The drawing under review shows one solid part. Ordinate dimensions are in mm from its lowest x, y, z. A direction names the side the tool comes from. Round coordinates to 2 decimals unless told otherwise and drop trailing zeros. Order: outer loops, then holes, each group sorted by start corner. A loop starts at its lowest first (then second) coordinate and runs counter-clockwise, first axis right, second up. Notation, with made-up numbers: (71.5, 64.5) - (120.5, 64.5) arc R26 ccw to (120.5, 99.5) - close; hole circle Ø1 at (57.25, 76). An arc over 180 degrees is marked (long way). One line per question, with ' | ' between items.
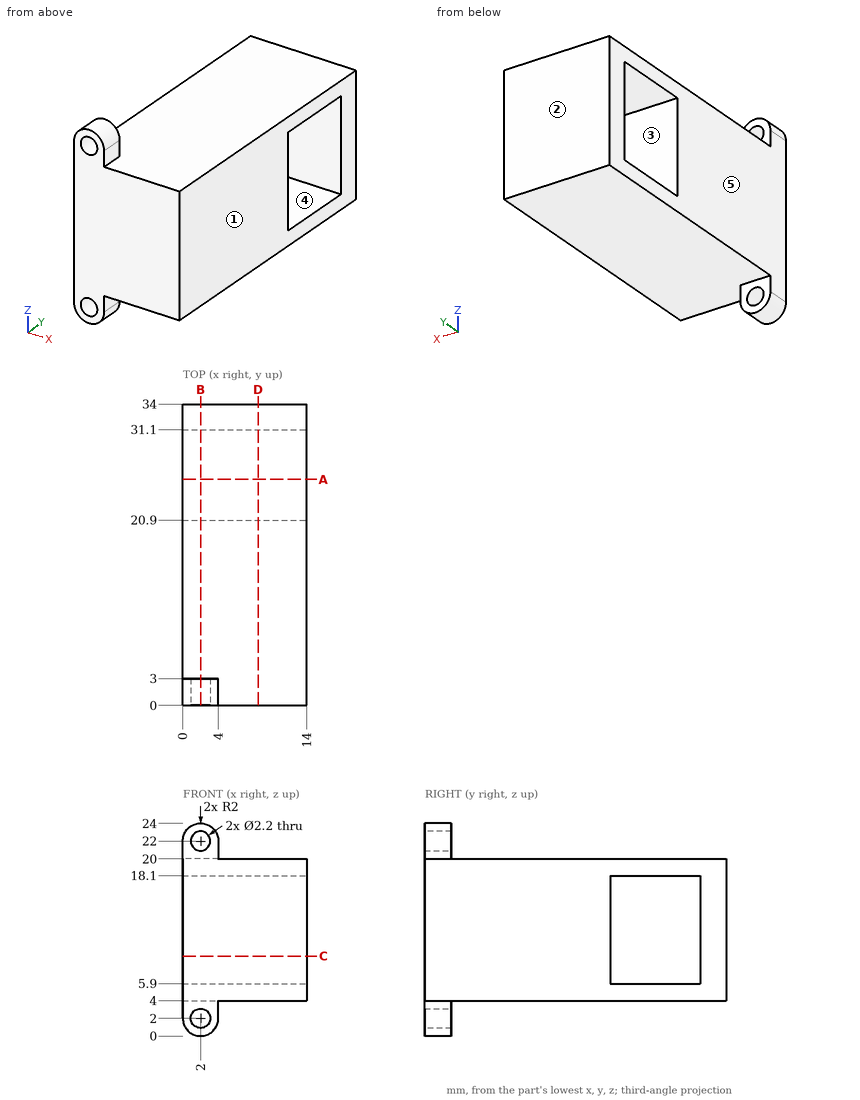
(1) We need section C-C on z = 9. State the section outline as (x, y) points.
Output values:
outline: (0, 0) - (14, 0) - (14, 20.9) - (0, 20.9) - close; (0, 31.1) - (14, 31.1) - (14, 34) - (0, 34) - close
(2) Insertion check: pin 1 (2 mm diameter, centred on x = 2.5, z = 2.5, fed in from +Y); pin 2 (0.6 mm diameter, centred on y = 2, z = 21, fed in from +X); pin 3 (1.5 mm diameter, centred on x = 5, y = 30.5, fed in from -Z); pin 4 (2.5 mm diameter, centred on x = 2, z = 2, fed in from -Y). Each pin has a flat end and moves straight along its axis. Give the tip position at first contact, or say it passes through.
Output values:
pin 1: y = 3 | pin 2: x = 4 | pin 3: z = 4 | pin 4: y = 0
(3) We need section D-D on x = 8.5. State the section outline as (y, z) points, plus the area to 3 significant figures.
Output values:
outline: (0, 4) - (34, 4) - (34, 20) - (0, 20) - close; hole (20.9, 5.9) - (31.1, 5.9) - (31.1, 18.1) - (20.9, 18.1) - close | area: 420 mm^2
(4) We need section A-A on y = 25.5. State the section outline as (x, z) points, plus the area to 3 significant figures.
Output values:
outline: (0, 4) - (14, 4) - (14, 5.9) - (0, 5.9) - close; (0, 18.1) - (14, 18.1) - (14, 20) - (0, 20) - close | area: 53.2 mm^2
(5) For probe 1 along Z at (x, y) = (13, 25.5); probe 2 along Y at (x, z) = (10.25, 14); probe 3 along X at (y, z) = (2.05, 22), list the stretches that pass through material, from the lowest coordinate up. Write a range as [from, to].
Output values:
probe 1: [4, 5.9], [18.1, 20] | probe 2: [0, 20.9], [31.1, 34] | probe 3: [0, 0.9], [3.1, 4]
(6) We need section B-B on x = 2. State the section outline as (y, z) points.
Output values:
outline: (0, 0) - (3, 0) - (3, 0.9) - (0, 0.9) - close; (0, 3.1) - (3, 3.1) - (3, 4) - (34, 4) - (34, 20) - (3, 20) - (3, 20.9) - (0, 20.9) - close; (0, 23.1) - (3, 23.1) - (3, 24) - (0, 24) - close; hole (20.9, 5.9) - (31.1, 5.9) - (31.1, 18.1) - (20.9, 18.1) - close
(7) For the marked faces 4 and 5, list the 3-axis set-ups (+Z, -Z, +X, -X, +Y, -Y) from which the entire face can be reached by the end or side of a thin tool; tool diameter is ignored.
Output values:
face 4: +X, -X | face 5: +Z, -Z, -X, +Y, -Y
(8) Mouldability with a two-part tool opening along Y and no side actions: class the marked faces 1, 2 and 3 as released by +Y, released by -Y, zero draft, split by the parting line, or undercut.
Output values:
face 1: zero draft | face 2: released by +Y | face 3: undercut
